Job drawing, mm, ordinate dimensions from the low corner. One solid piece. A direction names the side the tool comes from. Give positions to 0.01 mm unless a question says otherwise; leave off trailing zeros. Write each loop counter-clockwise with the first axis right and the second up, starting at its lowest first coordinate (ties: lowest second). Pieces come first, ordered by that corner, then holes. Notation, with made-up numbers: M 82,1 L 126,1 A20 ccw 126,24 Z; hole C 34,-12.5 d8. An arc over 180 degrees is marked long. Answer as CSV lines item,"result". Start each with the question number.
1) Slice it at B-B, the plane y = 12.5. Give the cut face in (x, z), plus the area to 3 significant figures.
2) Wall check: line 1 along Y through (x, z) = (1, 12.5); line 2 along Z through (x, y) = (2, 5.5) (1 decimal); line 3 along X through (y, z) = (22, 10.25). Give the ranges that are in metal, low to high. Write a range as from..to.
3) Slice it at C-C, the plane z = 12.5. Give the cut face in (x, y).
4) Pin check, flat tip, straight feed: pin 1 Ø4 at (x, y) = (9.5, 10.5) entering from +Z. Stop position of the tip, or through.
5) Slice it at D-D, the plane x = 8.5. Give the cut face in (y, z), plus the area to 3 significant figures.
6) Tool access for the marked faces 5 and 6: list every direction of +Z, -Z, +X, -X, +Y, -Y with a clear straight run to the whole face (end or side of a thin tool).
7) Mould opens along Y. For the marked faces 1, 2, 3 and 4 say: pulls with the +Y half, pulls with the -Y half, needs draft (parallel to the pull), parting line crosses it, or undercut.
8) Slice it at A-A, the plane x = 1. Give the cut face in (y, z), plus the area to 3 significant figures.
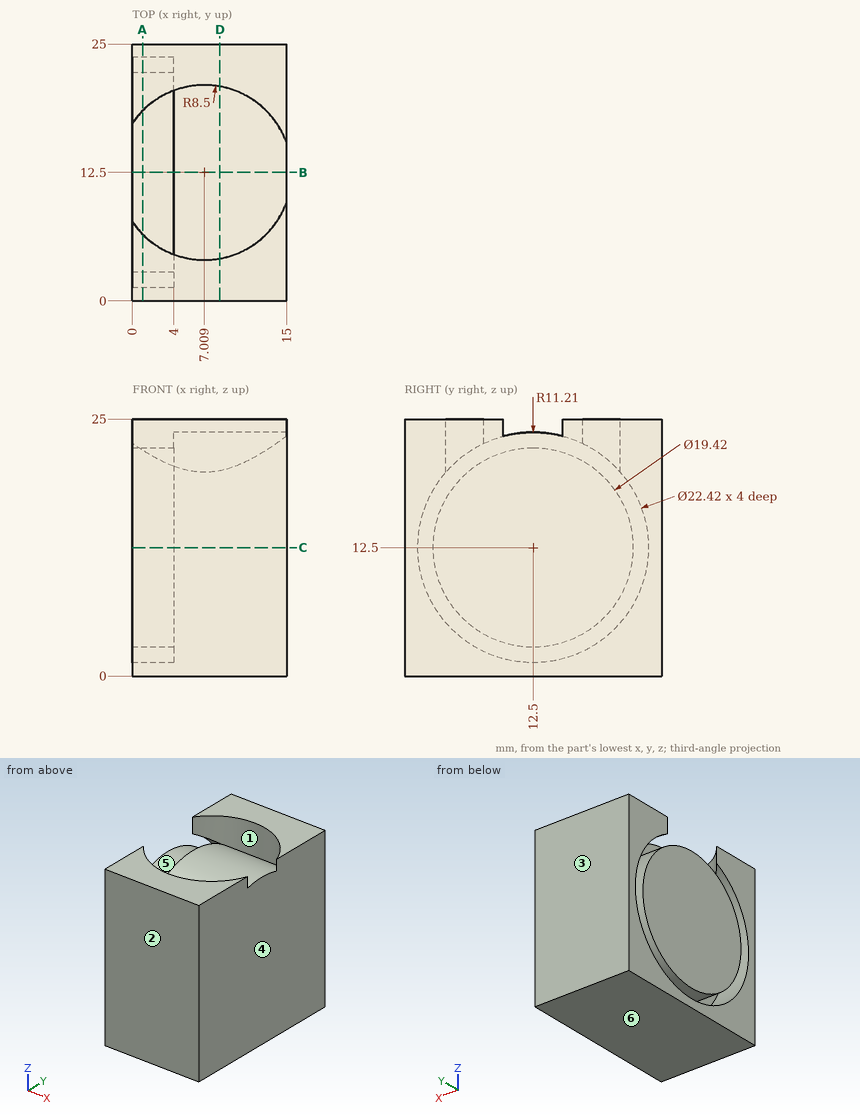
Found:
1,outline,"M 0,0 L 15,0 L 15,23.71 L 4,23.71 L 4,22.21 L 0,22.21 L 0,2.79 L 4,2.79 L 4,1.29 L 0,1.29 Z"
1,area,"344 mm²"
2,line 1,"0..1.29, 2.79..22.21, 23.71..25"
2,line 2,"0..3.7, 5.8..19.2, 21.3..25"
2,line 3,"4..15"
3,outline,"M 0,0 L 15,0 L 15,25 L 0,25 L 0,23.71 L 4,23.71 L 4,22.21 L 0,22.21 L 0,2.79 L 4,2.79 L 4,1.29 L 0,1.29 Z"
4,pin 1,"z = 23.71"
5,outline,"M 0,0 L 25,0 L 25,25 L 20.87,25 L 20.87,19.96 A11.21 ccw 4.13,19.96 L 4.13,25 L 0,25 Z"
5,area,"584 mm²"
6,face 5,"-X"
6,face 6,"-Z, +X, -X, +Y, -Y"
7,face 1,"undercut"
7,face 2,"pulls with the -Y half"
7,face 3,"pulls with the +Y half"
7,face 4,"needs draft"
8,outline,"M 0,0 L 25,0 L 25,25 L 18.51,25 L 18.51,21.96 A11.21 cw long 6.49,21.96 L 6.49,25 L 0,25 Z; C 12.5,12.5 d19.42"
8,area,"504 mm²"
